```python
from build123d import *

# Parameters (mm, degrees)
F0_W     = 60.075765
F0_H     = 27.85331
F1_DEPTH = 25.4
F2_R     = 7.011895
F2_R_2   = 7.03539
F3_DEPTH = 50.8
F4_R     = 10.314732
F5_DEPTH = 76.2


with BuildPart() as f1:
    # F0 (on Front) → F1 (new body)
    with BuildSketch(Plane.XZ):
        with Locations((6.007575, 1.092287)):
            Rectangle(F0_W, F0_H)
    extrude(amount=F1_DEPTH)

    # F2 (on face) → F3 (cut)
    with BuildSketch(Plane.XY.offset(15.018942)):
        with Locations((5.026927, -8.720485)):
            Circle(F2_R)
        with Locations((-12.451476, -8.720485)):
            Circle(F2_R_2)
    extrude(amount=-F3_DEPTH, mode=Mode.SUBTRACT)

    # F4 (on face) → F5 (join)
    with BuildSketch(Plane.XY.offset(15.018942)):
        with Locations((23.480423, -11.001698)):
            Circle(F4_R)
    extrude(amount=F5_DEPTH)


solid = f1.part
```
Design review of the part built by this model. Coordinates are the model's own, in mm. Give positions to 0.01 mm unless a question says otherwise; leave off trailing zeros. Write each loop counter-clockwise with the first axis right and the second up, starting at its lowest first coordinate (ties: lowest second). Pieces come first, ordered by that corner, then holes. Notation, with made-up numbers: (-25.5, -2.5) - (4.5, -2.5) arc R23 ccw to (4.5, 10.5) - close; hole circle Ø2 at (33, 67.5). An arc over 180 degrees is marked (long way). Return JSON: item names as keys, results as strings. Group by question number.
(1) To check wall thickness, follow probe 1 along Z at (x, y) = (-1.5, -4.5); probe 2 along Y at (x, z) = (-8.5, 3); probe 3 along X at (y, z) = (-3, 81). State the ranges of each line that lie inside material, in increasing order.
(2) We need section C-C, the plane x = 20.5. Give the boundary of the cut face in (y, z), then the cut area to 3 significant figures.
(3) Mouldability with a two-part tool opening along X and no side actions: class faces 1 (the flat face through (23, -11, 91.219)), 2 (the cylindrical face through (-8.67, -2.79, 1.29)), 3 (the cylindrical face through (33.319, -7.903, 52.586)), 4 (the cylindrical face through (11.715, -6.614, 1.287)) as +X half, -X half, draft (parallel to the pull), parting line (faces both ways), or undercut.
(4) We need section D-D, the plane z = 3.5. Give the boundary of the cut face in (x, y).
(5) We need section B-B, the plane x = -15. Give the boundary of the cut face in (y, z).
(6) Insertion check: pin 1 (12 mm diameter, centred on x = 7.5, y = -8, fed in from +Z); pin 2 (10 mm diameter, centred on x = -7.5, y = -3, fed in from +Z); pin 3 (2 mm diameter, centred on y = -15, z = 41, fed in from -X); pin 4 (1 mm diameter, centred on x = 19.5, z = 48.5, fed in from -Y). Each pin has a flat end and moves straight along its axis. Give the tip position at first contact, or say it passes through.
(7) We need section A-A, the plane y = -14.5. Give the boundary of the cut face in (x, z).
Reported:
{
 "1": {"probe 1": "z = -12.83 to 15.02", "probe 2": "y = -25.4 to -14.54, -2.9 to 0", "probe 3": "x = 16.97 to 29.99"},
 "2": {"outline": "(-25.4, -12.83) - (0, -12.83) - (0, 15.02) - (-1.13, 15.02) - (-1.13, 91.22) - (-20.88, 91.22) - (-20.88, 15.02) - (-25.4, 15.02) - close", "area": "2,210 mm2"},
 "3": {"face 1": "draft", "face 2": "undercut", "face 3": "parting line", "face 4": "undercut"},
 "4": {"outline": "(-24.03, -25.4) - (36.05, -25.4) - (36.05, 0) - (-24.03, 0) - close; hole circle Ø14.07 at (-12.45, -8.72); hole circle Ø14.02 at (5.03, -8.72)"},
 "5": {"outline": "(-25.4, -12.83) - (-15.28, -12.83) - (-15.28, 15.02) - (-25.4, 15.02) - close; (-2.16, -12.83) - (0, -12.83) - (0, 15.02) - (-2.16, 15.02) - close"},
 "6": {"pin 1": "stops at z = 91.22", "pin 2": "stops at z = 15.02", "pin 3": "stops at x = 13.61", "pin 4": "stops at y = -20.71"},
 "7": {"outline": "(-24.03, -12.83) - (-16.46, -12.83) - (-16.46, 15.02) - (-24.03, 15.02) - close; (-8.44, -12.83) - (1.06, -12.83) - (1.06, 15.02) - (-8.44, 15.02) - close; (9, -12.83) - (36.05, -12.83) - (36.05, 15.02) - (33.18, 15.02) - (33.18, 91.22) - (13.78, 91.22) - (13.78, 15.02) - (9, 15.02) - close"}
}
